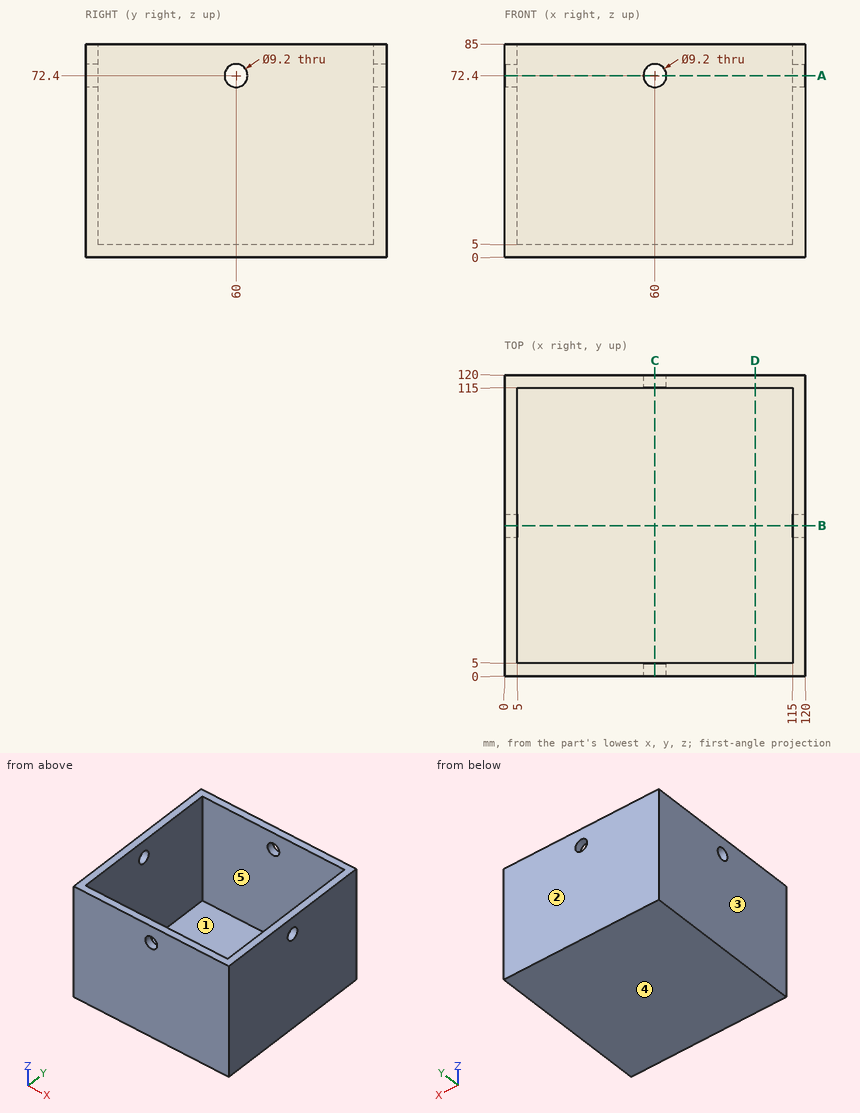
Design review of the part shown in the three views and the two pictorial views. Dimensions are in mm from the part's minimum x, y and z. A direction names the side the tool comes from. Coordinates: 2 decimals unless noted, no trailing zeros. Write each loop counter-clockwise with the first axis right and the second up, starting at its lowest first coordinate (ties: lowest second). Pieces come first, ordered by that corner, then holes. Notation, with made-up numbers: (-37, -22.5) - (-27, -22.5) arc R24 ccw to (-27, 14.5) - close; hole circle Ø4 at (39.25, 62.25). An arc over 180 degrees is marked (long way). Write item = value, one per line.
(1) For line 1 (X direction, y = 100.5, z = 9.5); line 2 (Y direction, x = 117.45, z = 72.4), list the stretches that pass through material, from the lowest coordinate up. Write a range as [from, to].
Result sheet:
line_1 = [0, 5], [115, 120]
line_2 = [0, 55.4], [64.6, 120]
(2) Consider section A-A, the plane z = 72.4. Give the boundary of the cut face in (x, y), then the cut area to 3 significant figures.
Result sheet:
outline = (0, 0) - (55.4, 0) - (55.4, 5) - (5, 5) - (5, 55.4) - (0, 55.4) - close; (0, 64.6) - (5, 64.6) - (5, 115) - (55.4, 115) - (55.4, 120) - (0, 120) - close; (64.6, 0) - (120, 0) - (120, 55.4) - (115, 55.4) - (115, 5) - (64.6, 5) - close; (64.6, 115) - (115, 115) - (115, 64.6) - (120, 64.6) - (120, 120) - (64.6, 120) - close
area = 2,120 mm^2
(3) Mouldability with a two-part tool opening along X and no side actions: class the marked faces 3, 4 and 5 as pulls with the +X half, pulls with the -X half, needs draft (parallel to the pull), parting line crosses it, or undercut.
Result sheet:
face_3 = pulls with the -X half
face_4 = needs draft
face_5 = undercut
(4) Consider section D-D, the plane x = 100. Give the boundary of the cut face in (y, z), then the cut area to 3 significant figures.
Result sheet:
outline = (0, 0) - (120, 0) - (120, 85) - (115, 85) - (115, 5) - (5, 5) - (5, 85) - (0, 85) - close
area = 1,400 mm^2
(5) Consider section B-B, the plane y = 60. Give the boundary of the cut face in (x, z).
Result sheet:
outline = (0, 0) - (120, 0) - (120, 67.8) - (115, 67.8) - (115, 5) - (5, 5) - (5, 67.8) - (0, 67.8) - close; (0, 77) - (5, 77) - (5, 85) - (0, 85) - close; (115, 77) - (120, 77) - (120, 85) - (115, 85) - close
(6) For P1, Ø2, axis at x = 24.5, y = 93.5, coming from the -Z side, flat-tipped, find the tip position at first contact; note if it passes through.
Result sheet:
P1 = 0
(7) Machinability: for the marked faces 1 and 2, which of the approach directions +Z, -Z, +X, -X, +Y, -Y give a long, thin tool a straight path to every point of the face, cutting with its end or side? Answer none if there is none.
Result sheet:
face_1 = +Z
face_2 = +Z, -Z, +X, -X, +Y
